Geometry check sheet. Reference: the model listing, model coordinates, mm. A direction names the side the tool comes from. Give positions to 0.01 mm unless a question says otherwise; leave off trailing zeros. Write each loop counter-clockwise with the first axis right and the second up, starting at its lowest first coordinate (ties: lowest second). Pieces come first, ordered by that corner, then holes. Notation, with made-up numbers: (-38, -26.5) - (-26, -26.5) arc R15 cw to (-26, -10.5) - close; hole circle Ø3 at (73, 17). An arc over 180 degrees is marked (long way). One line per question, with ' | ' between items. Start each with the question number.
Q1. Set-up check for faces 1 (the face through (-1, 12, 0)), 2 (the face through (79, 0, 16)), 3 (the face through (-79, 0, 16)): record each of +Z, -Z, +X, -X, +Y, -Y from which the full face is reachable in a straight line by a thin tool's end or side.
Q2. Section check B-B on y = 6. Record the boundary of the cut face in (x, z), and give its area (3 significant figures).
Q3. Gauge pin test, flat ends, axial feed: P1, Ø10, axis at x = -20.5, z = 3, coming from the +Y side; P2, Ø10, axis at x = 43, z = 16, coming from the -Y side; P3, Ø2.5, axis at x = 79.5, z = 16.5, coming from the -Y side. Record the tip position at first contact, or that the pin passes through.
Q4. Release check for a two-part mould opening along X. For faces 4 (the face through (-1, 12, 31.75)), 5 (the face through (80.962, 2, 16)), 6 (the face through (-43.93, -3.26, 15.65)) record: +X half, -X half, draft (parallel to the pull), parting line (faces both ways), or undercut.
Q5. Thickness scan on L1, parallel to Y at x = 0, z = 9.5; L2, parallel to X at y = -0.5, z = 15.5; L3, parallel to Y at x = -4.5, z = 28. Record the ranges inside material, lowest first. Write a range as [from, to].
Q6. Section check D-D on x = 24. Record the boundary of the cut face in (y, z), and give its area (3 significant figures).
Q7. Section check A-A on x = 0. Record the boundary of the cut face in (y, z), and give its area (3 significant figures).
Q8. Section check C-C on y = -1.5. Record the boundary of the cut face in (x, z), and give its area (3 significant figures).
```python
from build123d import *

# Parameters (mm, degrees)
F0_W     = 3.175
F0_H     = 3.175
F1_DEPTH = 31.75
F2_R     = 11.1125
F3_DEPTH = 31.75
F4_R     = 19.05
F5_R     = 19.05


with BuildPart() as f1:
    # F0 (on Top) → F1 (new body)
    with BuildSketch(Plane.XY):
        with BuildLine():
            ThreePointArc((15.475885, -13.652963), (19.304015, -7.298042), (20.6375, 0))
            ThreePointArc((20.6375, 0), (16.81923, 11.959093), (6.777302, 19.492937))
            ThreePointArc((6.777302, 19.492937), (-5.238574, 19.961557), (-15.475885, 13.652963))
            ThreePointArc((-15.475885, 13.652963), (-19.961557, -5.238574), (-6.777302, -19.492937))
            ThreePointArc((-6.777302, -19.492937), (5.238574, -19.961557), (15.475885, -13.652963))
        make_face()
        with BuildLine():
            ThreePointArc((6.777302, 19.492937), (16.81923, 11.959093), (20.6375, 0))
            ThreePointArc((20.6375, 0), (19.304015, -7.298042), (15.475885, -13.652963))
            ThreePointArc((15.475885, -13.652963), (44.398982, 3.363524), (77.7875, 0))
            Line((77.7875, 0), (77.7875, 3.175))
            Line((77.7875, 3.175), (80.9625, 3.175))
            ThreePointArc((80.9625, 3.175), (46.643898, 23.945214), (6.777302, 19.492937))
        make_face()
        with BuildLine():
            ThreePointArc((-6.777302, -19.492937), (-19.961557, -5.238574), (-15.475885, 13.652963))
            ThreePointArc((-15.475885, 13.652963), (-44.398982, -3.363524), (-77.7875, 0))
            Line((-77.7875, 0), (-77.7875, -3.175))
            Line((-77.7875, -3.175), (-80.9625, -3.175))
            ThreePointArc((-80.9625, -3.175), (-46.643898, -23.945214), (-6.777302, -19.492937))
        make_face()
        with Locations((79.375, 1.5875)):
            Rectangle(F0_W, F0_H)
        with Locations((-79.375, -1.5875)):
            Rectangle(F0_W, F0_H)
    extrude(amount=F1_DEPTH)

    # F2 (on Top) → F3 (cut)
    with BuildSketch(Plane.XY):
        Circle(F2_R)
    extrude(amount=F3_DEPTH, mode=Mode.SUBTRACT)

    # F4
    f4_edges = [f1.edges().sort_by_distance(p)[0] for p in [
        (-6.777302, -19.492937, 15.875),
    ]]
    fillet(f4_edges, radius=F4_R)

    # F5
    f5_edges = [f1.edges().sort_by_distance(p)[0] for p in [
        (6.777302, 19.492937, 15.875),
    ]]
    fillet(f5_edges, radius=F5_R)


solid = f1.part
```
Working result:
1) face 1: -Z, +X, -X, +Y, -Y | face 2: +Z, -Z, +X, -Y | face 3: +Z, -Z, -X, +Y
2) outline: (-23.81, 0) - (-9.35, 0) - (-9.35, 31.75) - (-23.81, 31.75) - close; (9.35, 0) - (78.44, 0) - (78.44, 31.75) - (9.35, 31.75) - close | area: 2,650 mm2
3) P1: stops at y = 13.63 | P2: stops at y = 1.54 | P3: stops at y = 0
4) face 4: draft | face 5: +X half | face 6: undercut
5) L1: y = [-20.64, -11.11], [11.11, 20.64] | L2: x = [-80.96, -76.62], [-35.28, -11.1], [11.1, 33.02] | L3: y = [-20.33, -10.16], [10.16, 20.14]
6) outline: (-5.86, 0) - (24.71, 0) - (24.71, 31.75) - (-5.86, 31.75) - close | area: 971 mm2
7) outline: (-20.64, 0) - (-11.11, 0) - (-11.11, 31.75) - (-20.64, 31.75) - close; (11.11, 0) - (20.64, 0) - (20.64, 31.75) - (11.11, 31.75) - close | area: 605 mm2
8) outline: (-80.96, 0) - (-74.02, 0) - (-74.02, 31.75) - (-80.96, 31.75) - close; (-37.88, 0) - (-11.01, 0) - (-11.01, 31.75) - (-37.88, 31.75) - close; (11.01, 0) - (31, 0) - (31, 31.75) - (11.01, 31.75) - close | area: 1,710 mm2
